from build123d import *

# Parameters (mm, degrees)
SKETCH_1_W      = 30
SKETCH_1_H      = 30
EXTRUDE_1_DEPTH = 3.3
SKETCH_2_R      = 0.3
EXTRUDE_2_DEPTH = 10


with BuildPart() as part:
    # 草图1 → 拉伸1 (new body)
    with BuildSketch(Plane(origin=(0, 0, 0), x_dir=(1, 0, 0), z_dir=(0, 1, 0))):
        Rectangle(SKETCH_1_W, SKETCH_1_H)
    extrude(amount=EXTRUDE_1_DEPTH)

    # 草图2 → 拉伸2 (add)
    with BuildSketch(Plane.XY.offset(15)):
        with Locations(Location((-12, 1.65, 0), (0, 0, 180))):
            Circle(SKETCH_2_R)
        with Locations(Location((12, 1.65, 0), (0, 0, 180))):
            Circle(SKETCH_2_R)
    extrude(amount=EXTRUDE_2_DEPTH)


solid = part.part
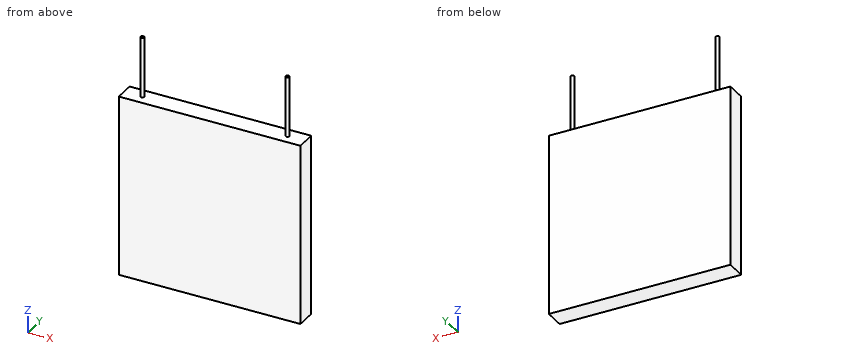
Check sheet for the modelled part. Datum: model origin and axes. Units: mm. Coordinates: 2 decimals unless noted, no trailing zeros. Write each loop counter-clockwise with the first axis right and the second up, starting at its lowest first coordinate (ties: lowest second). Pieces come first, ordered by that corner, then holes.
Item 1: Scan line: probe 1 along Z at (x, y) = (2.25, 3.05). Record every from-to range of solid material in increasing order.
Numbers:
probe 1: z = -15 to 15
Item 2: Cross-section at A-A on z = 17.5. Record the boundary of the cut face in (x, y), then the cut area to 3 significant figures.
Numbers:
outline: circle Ø0.6 at (-12, 1.65); circle Ø0.6 at (12, 1.65)
area: 0.565 mm2
Item 3: Cross-section at C-C on x = 5.5. Record the boundary of the cut face in (y, z), then the cut area to 3 significant figures.
Numbers:
outline: (0, -15) - (3.3, -15) - (3.3, 15) - (0, 15) - close
area: 99.0 mm2
Item 4: Cross-section at B-B on y = 0.5. Record the boundary of the cut face in (x, z).
Numbers:
outline: (-15, -15) - (15, -15) - (15, 15) - (-15, 15) - close
